The listing builds one solid part. Answer for the finished solid, in the listing's coordinates (mm). A direction names the side the tool comes from. Give positions to 0.01 mm unless a question says otherwise; leave off trailing zeros. Loops run counter-clockwise (first coordinate to the right, second up) from the corner with the lowest first, then second, coordinate; pieces in that order, holes last. Notation, with made-up numbers: M 32.5,-11 L 90.5,-11 A28 cw 90.5,13 Z; hole C -37,-11.5 d2. An arc over 180 degrees is marked long. Use one line per item in the form item = value. Start each with the question number.
1. The part is cut by section A-A (y = -21.5). Write down the section's boundary in (x, z), and give its area (3 significant figures).
2. The part is cut by section D-D (x = 32.5). Write down the section's boundary in (y, z).
3. The part is cut by section B-B (z = -4.5). Write down the section's boundary in (x, y), and give its area (3 significant figures).
4. The part is cut by section C-C (z = -18.5). Write down the section's boundary in (x, y), and give its area (3 significant figures).
5. Each of these flat-tipped pins is pushed along its axis until it touches: pin 1 Ø3.5 at (y, z) = (-11.62, -37.99) entering from -X; pin 2 Ø11.5 at (y, z) = (-13.5, -25.5) entering from +X; pin 3 Ø13.5 at (x, y) = (82.5, -5) entering from -Z; pin 4 Ø7.5 at (y, z) = (2.5, 20.5) entering from +X. Where does it stop, or does it pass through?
6. For faces 4 (the face through (95, 1, 0)), 5 (the face through (65, -18.9, -36.5)), 6 (the face through (7, -19, 0)), 7 (the face through (72, -38.25, -25)), 8 (the face through (125, -10, -31)), determine the directions among +Z, -Z, +X, -X, +Y, -Y from which every point of the face is accessible in a straight line to the end or side of a thin tool.
7. The mould has two halves that part along X. Classify faces 1 (the face through (40, 3, -70)), 2 (the face through (147, 0, -25)), 3 (the face through (80, -18.9, -36.5)): released by +X, released by -X, zero draft, split by the parting line, or undercut.
8. Straight lines are drawn through the part: line 1 (X direction, y = -6, z = -28.5); line 2 (Y direction, x = 122.2, z = -25) (3 decimals); line 3 (Z direction, x = 8.5, y = -9.5). For each, find the intervals that lie inside material, in ascending order. Write a range as from..to.
from build123d import *

# Parameters (mm, degrees)
BOSS_EXTRUDE2_DEPTH = 7
SKETCH2_W           = 15
SKETCH2_H           = 50
SKETCH2_W_2         = 5
BOSS_EXTRUDE4_DEPTH = 38.25
SKETCH10_R          = 11
CUT_EXTRUDE5_DEPTH  = 15
SKETCH11_R          = 11
CUT_EXTRUDE7_DEPTH  = 15
SKETCH23_R          = 10
SKETCH23_R_2        = 1.5
CUT_EXTRUDE10_DEPTH = 5
SKETCH12_R          = 10
SKETCH12_R_2        = 1.5
CUT_EXTRUDE9_DEPTH  = 5


with BuildPart() as part:
    # Sketch1 → Boss-Extrude2 (new body)
    with BuildSketch(Plane(origin=(0, 0, 0), x_dir=(1, 0, 0), z_dir=(0, 1, 0))):
        Polygon((40, 0), (170, 0), (170, 50), (40, 50), (40, 90), (0, 90), (0, 50), (0, 0), (0, -40), (40, -40), align=None)
    extrude(amount=BOSS_EXTRUDE2_DEPTH)

    # Sketch2 → Boss-Extrude4 (add)
    with BuildSketch(Plane.XZ):
        with Locations((7.5, -25)):
            Rectangle(SKETCH2_W, SKETCH2_H)
        with Locations((72.5, -25)):
            Rectangle(SKETCH2_W, SKETCH2_H)
        with Locations((122.5, -25)):
            Rectangle(SKETCH2_W_2, SKETCH2_H)
    extrude(amount=BOSS_EXTRUDE4_DEPTH)

    # Sketch10 → Cut-Extrude5 (cut)
    with BuildSketch(Plane.ZY):
        with Locations((-25, -19.125)):
            Circle(SKETCH10_R)
    extrude(amount=-CUT_EXTRUDE5_DEPTH, mode=Mode.SUBTRACT)

    # Sketch11 → Cut-Extrude7 (cut)
    with BuildSketch(Plane.ZY.offset(-65)):
        with Locations((-25, -19.125)):
            Circle(SKETCH11_R)
    extrude(amount=-CUT_EXTRUDE7_DEPTH, mode=Mode.SUBTRACT)

    # Sketch23 → Cut-Extrude10 (cut)
    with BuildSketch(Plane(origin=(125, 0, 0), x_dir=(0, 0, -1), z_dir=(1, 0, 0))):
        with Locations((25, -19.125)):
            Circle(SKETCH23_R)
        with Locations((12.009618943, -11.625)):
            Circle(SKETCH23_R_2)
        with Locations((37.990381057, -11.625)):
            Circle(SKETCH23_R_2)
        with Locations((25, -34.125)):
            Circle(SKETCH23_R_2)
    extrude(amount=-CUT_EXTRUDE10_DEPTH, mode=Mode.SUBTRACT)

    # Sketch12 → Cut-Extrude9 (cut)
    with BuildSketch(Plane(origin=(125, 0, 0), x_dir=(0, 0, -1), z_dir=(1, 0, 0))):
        with Locations((25, -19.125)):
            Circle(SKETCH12_R)
        with Locations((12.009618943, -11.625)):
            Circle(SKETCH12_R_2)
        with Locations((37.990381057, -11.625)):
            Circle(SKETCH12_R_2)
        with Locations((25, -34.125)):
            Circle(SKETCH12_R_2)
    extrude(amount=-CUT_EXTRUDE9_DEPTH, mode=Mode.SUBTRACT)


solid = part.part
Derived:
q1.outline = M 0,-50 L 15,-50 L 15,-35.74 L 0,-35.74 Z; M 0,-14.26 L 15,-14.26 L 15,0 L 0,0 Z; M 65,-50 L 80,-50 L 80,-35.74 L 65,-35.74 Z; M 65,-14.26 L 80,-14.26 L 80,0 L 65,0 Z; M 120,-50 L 125,-50 L 125,-34.71 L 120,-34.71 Z; M 120,-15.29 L 125,-15.29 L 125,0 L 120,0 Z
q1.area = 1,010 mm2
q2.outline = M 0,-90 L 7,-90 L 7,40 L 0,40 Z
q3.outline = M 0,-38.25 L 15,-38.25 L 15,0 L 65,0 L 65,-38.25 L 80,-38.25 L 80,0 L 120,0 L 120,-38.25 L 125,-38.25 L 125,0 L 170,0 L 170,7 L 0,7 Z
q3.area = 2,530 mm2
q4.outline = M 0,-38.25 L 15,-38.25 L 15,-28 L 0,-28 Z; M 0,-10.25 L 15,-10.25 L 15,0 L 65,0 L 65,-10.25 L 80,-10.25 L 80,0 L 120,0 L 120,-11.53 L 125,-11.53 L 125,0 L 170,0 L 170,7 L 0,7 Z; M 65,-38.25 L 80,-38.25 L 80,-28 L 65,-28 Z; M 120,-38.25 L 125,-38.25 L 125,-26.72 L 120,-26.72 Z
q4.area = 1,920 mm2
q5.pin_1 = 0
q5.pin_2 = 125
q5.pin_3 = -50
q5.pin_4 = 40
q6.face_4 = +Z, +X, +Y, -Y
q6.face_5 = +Z, -Z, -Y
q6.face_6 = +Z, +X, -X, -Y
q6.face_7 = +Z, -Z, +X, -X, -Y
q6.face_8 = +Z, -Z, +X, -Y
q7.face_1 = released by +X
q7.face_2 = zero draft
q7.face_3 = undercut
q8.line_1 = 0..15, 65..80, 120..125
q8.line_2 = -38.25..-35.625, -32.625..-29.125, -9.125..7
q8.line_3 = -50..-30.33, -19.67..0
